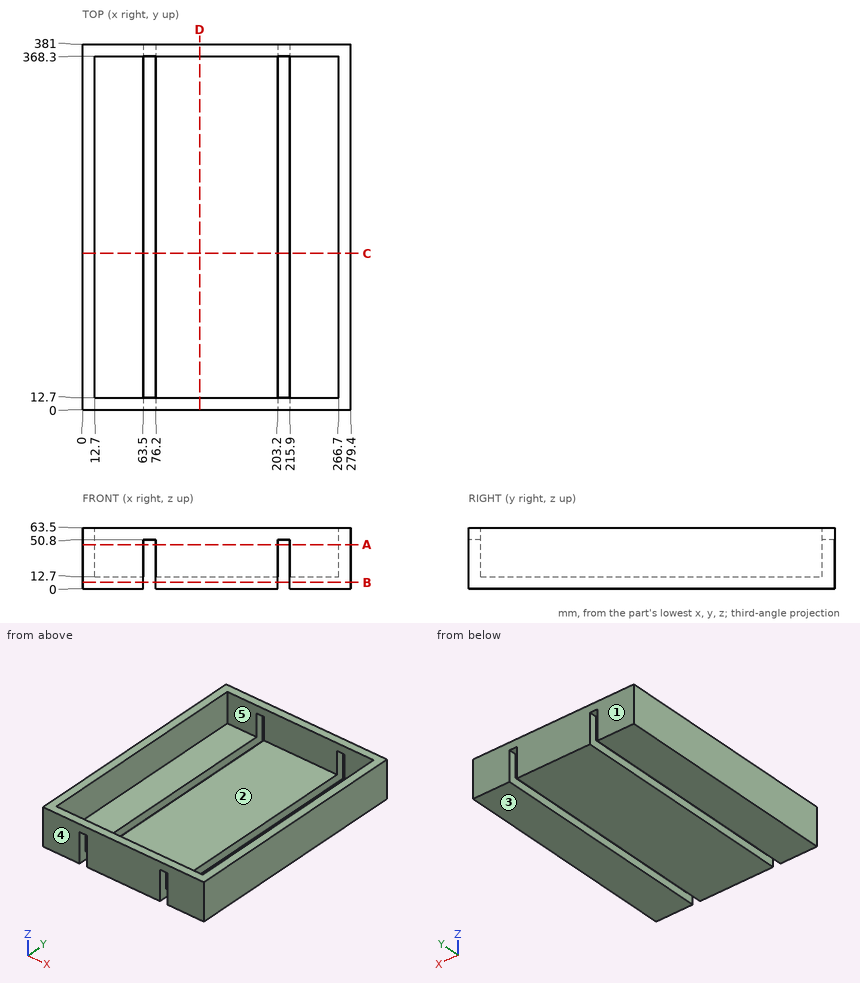
Part print with two shaded views. Sizes in mm from the minimum x, y, z corner. A direction names the side the tool comes from. Round coordinates to 2 decimals unless told otherwise and drop trailing zeros. Loops run counter-clockwise (first coordinate to the right, second up) from the corner with the lowest first, then second, coordinate; pieces in that order, holes last.
1. Drill centre lines: line 1 along X through (y, z) = (253.5, 11.5); line 2 along Y through (x, z) = (61, 61); line 3 along X through (y, z) = (243, 26.5). Where is each one in solid material? Low to high.
Solutions:
line 1: x = 0 to 63.5, 76.2 to 203.2, 215.9 to 279.4
line 2: y = 0 to 12.7, 368.3 to 381
line 3: x = 0 to 12.7, 266.7 to 279.4
2. Slice it at B-B (z = 6.5). Give the cut face in (x, y).
Solutions:
outline: (0, 0) - (63.5, 0) - (63.5, 381) - (0, 381) - close; (76.2, 0) - (203.2, 0) - (203.2, 381) - (76.2, 381) - close; (215.9, 0) - (279.4, 0) - (279.4, 381) - (215.9, 381) - close
3. Slice it at C-C (y = 163). Give the cut face in (x, z).
Solutions:
outline: (0, 0) - (63.5, 0) - (63.5, 12.7) - (12.7, 12.7) - (12.7, 63.5) - (0, 63.5) - close; (76.2, 0) - (203.2, 0) - (203.2, 12.7) - (76.2, 12.7) - close; (215.9, 0) - (279.4, 0) - (279.4, 63.5) - (266.7, 63.5) - (266.7, 12.7) - (215.9, 12.7) - close
4. 3-axis set-ups, long thin cutter, end or side, ignore diameter. For the marked faces 1 and 2: which of +Z, -Z, +X, -X, +Y, -Y reach the whole face in a straight line?
Solutions:
face 1: +Z, -Z, +X, -X, +Y
face 2: +Z
5. Slice it at A-A (z = 46). Give the cut face in (x, y), and give its area (3 significant figures).
Solutions:
outline: (0, 0) - (63.5, 0) - (63.5, 12.7) - (12.7, 12.7) - (12.7, 368.3) - (63.5, 368.3) - (63.5, 381) - (0, 381) - close; (76.2, 0) - (203.2, 0) - (203.2, 12.7) - (76.2, 12.7) - close; (76.2, 368.3) - (203.2, 368.3) - (203.2, 381) - (76.2, 381) - close; (215.9, 0) - (279.4, 0) - (279.4, 381) - (215.9, 381) - (215.9, 368.3) - (266.7, 368.3) - (266.7, 12.7) - (215.9, 12.7) - close
area: 15,500 mm2
6. Slice it at D-D (x = 122). Give the cut face in (y, z).
Solutions:
outline: (0, 0) - (381, 0) - (381, 63.5) - (368.3, 63.5) - (368.3, 12.7) - (12.7, 12.7) - (12.7, 63.5) - (0, 63.5) - close
7. Two-plate mould, pull along Y, no slides. Class the marked faces 3, 4 and 5: pulls with the +Y half, pulls with the -Y half, needs draft (parallel to the pull), parting line crosses it, or undercut.
Solutions:
face 3: needs draft
face 4: pulls with the -Y half
face 5: undercut
8. Flat gauge pins, fed straight in: pin 1 (10 mm diameter, centred on x = 209, y = 377.5, fed in from -Z); pin 2 (15 mm diameter, centred on x = 43, y = 251, fed in from +Z). Where does each tip first touch, or does it go through?
Solutions:
pin 1: stops at z = 50.8
pin 2: stops at z = 12.7
